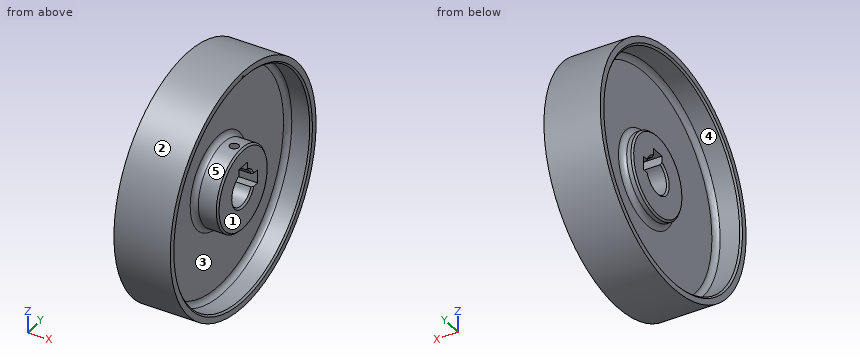
```python
from build123d import *

# Parameters (mm, degrees)
F2_R     = 3
F4_DEPTH = 25
F5_SIZE  = 1
F9_D     = 5.1054
F9_DEPTH = 56.7408363237


with BuildPart() as f1:
    # F0 (on Front) → F1 (revolve)
    with BuildSketch(Plane.XZ):
        Polygon((-11.987469025, 24.25), (-11.987469025, 0), (12.012530975, 0), (12.012530975, 24.25), (-2.487469025, 24.25), (-2.487469025, 65.9), (12.012530975, 65.9), (12.012530975, 70.4), (-20.987469025, 70.4), (-20.987469025, 65.9), (-5.487469025, 65.9), (-5.487469025, 24.25), align=None)
    revolve(axis=Axis((-25.877635926, 0, 0), (-1, 0, 0)))

    # F2
    f2_edges = [f1.edges().sort_by_distance(p)[0] for p in [
        (-2.487469, 0, -24.25),
        (-2.487469, 0, -65.9),
        (-5.487469, 0, -24.25),
        (-5.487469, 0, -65.9),
    ]]
    fillet(f2_edges, radius=F2_R)

    # F3 (on face) → F4 (cut)
    with BuildSketch(Plane.YZ.offset(12.012530975)):
        with BuildLine():
            Line((-4, 14), (-4, 9.1651513899))
            ThreePointArc((-4, 9.1651513899), (-7.0710678119, -7.0710678119), (9.1651513899, -4))
            Line((9.1651513899, -4), (14, -4))
            Line((14, -4), (14, 4))
            Line((14, 4), (9.1651513899, 4))
            ThreePointArc((9.1651513899, 4), (7.0710678119, 7.0710678119), (4, 9.1651513899))
            Line((4, 9.1651513899), (4, 14))
            Line((4, 14), (-4, 14))
        make_face()
    extrude(amount=-F4_DEPTH, mode=Mode.SUBTRACT)

    # F5
    f5_edges = [f1.edges().sort_by_distance(p)[0] for p in [
        (12.012531, 0, -65.9),
        (12.012531, 0, -24.25),
        (12.012531, -7.071068, -7.071068),
        (12.012531, 7.071068, 7.071068),
        (-11.987469, 0, -24.25),
        (-20.987469, 0, -65.9),
        (-11.987469, -7.071068, -7.071068),
        (-11.987469, 7.071068, 7.071068),
    ]]
    chamfer(f5_edges, length=F5_SIZE)

    # F9 (through all, one way)
    with BuildSketch(Plane(origin=(2.5485619967, 0, 14.4536133183), x_dir=(0.984807753, 0, -0.1736481777), z_dir=(-0.1736481777, 0, -0.984807753))):
        with Locations((2.532057697, 0)):
            Circle(F9_D / 2)
    extrude(amount=-F9_DEPTH, mode=Mode.SUBTRACT)


solid = f1.part
```
Input: part model. Units: mm. Frame: model coordinates. Face numbers are marked on the shaded views. A direction names the side the tool comes from. Give positions to 0.01 mm unless a question says otherwise; leave off trailing zeros. Write item = value, one per line. Start each with the question number.
1) Pin query (flat end, axial travel): pin 1 (5.5 mm diameter, centred on x = -5.5, y = 11.5, fed in from +Z); pin 2 (9 mm diameter, centred on x = -3.5, z = 1.5, fed in from -Y); pin 3 (12 mm diameter, centred on x = -2.5, z = -26.5, fed in from +Y); pin 4 (6.5 mm diameter, centred on x = -0.5, y = -0.5, fed in from -Z). Return the tip coordinate at first contact, or that it passes through.
2) Material intervals for L1, parallel to Y at x = 8, z = 0; L2, parallel to Y at x = -14.75, z = 0; L3, parallel to Z at x = -7, y = 5, sorted ascending. Write a range as [from, to].
3) Reachability of the marked faces 4 and 5 from +Z, -Z, +X, -X, +Y, -Y: full face, straight path, thin tool, end or side. Return the list, or none.
4) Draft query along Y for the marked faces 1, 2 and 3. Return one class per face: pulls with the +Y half, pulls with the -Y half, needs draft (parallel to the pull), parting line crosses it, or undercut.
Answers follow:
q1.pin_1 = 69.85
q1.pin_2 = -70.4
q1.pin_3 = 67.35
q1.pin_4 = -70.4
q2.L1 = [-70.4, -65.9], [-24.25, -10], [14, 24.25], [65.9, 70.4]
q2.L2 = [-70.4, -65.9], [65.9, 70.4]
q2.L3 = [-70.22, -65.31], [-24.13, -8.66], [8.66, 24.13], [65.31, 70.22]
q3.face_4 = -X
q3.face_5 = +X
q4.face_1 = needs draft
q4.face_2 = parting line crosses it
q4.face_3 = undercut
